Geometry check sheet. Reference: the model listing, model coordinates, mm. Face numbers are marked on the shaded views. A direction names the side the tool comes from. Round coordinates to 2 decimals unless told otherwise and drop trailing zeros. Write each loop counter-clockwise with the first axis right and the second up, starting at its lowest first coordinate (ties: lowest second). Pieces come first, ordered by that corner, then holes.
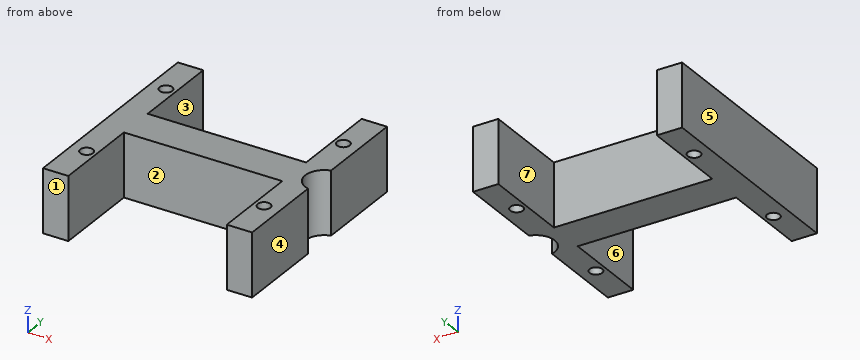
from build123d import *

# Parameters (mm, degrees)
CYLINDER156_R     = 3
CYLINDER156_DEPTH = 20
CYLINDER107_R     = 1
CYLINDER107_DEPTH = 15
CYLINDER108_R     = 1
CYLINDER108_DEPTH = 15
CYLINDER106_R     = 1
CYLINDER106_DEPTH = 15
CYLINDER105_R     = 1
CYLINDER105_DEPTH = 15
PAD005_DEPTH      = 10


with BuildPart() as zylinder156:
    # Cylinder156 → Cylinder156 (new body)
    with BuildSketch(Plane(origin=(28.75, 0, -21), x_dir=(1, 0, 0), z_dir=(0, 0, 1))):
        Circle(CYLINDER156_R)
    extrude(amount=CYLINDER156_DEPTH)


with BuildPart() as zylinder107:
    # Cylinder107 → Cylinder107 (new body)
    with BuildSketch(Plane(origin=(25.5, -10, -20), x_dir=(1, 0, 0), z_dir=(0, 0, 1))):
        Circle(CYLINDER107_R)
    extrude(amount=CYLINDER107_DEPTH)


with BuildPart() as zylinder108:
    # Cylinder108 → Cylinder108 (new body)
    with BuildSketch(Plane(origin=(25.5, 10, -20), x_dir=(1, 0, 0), z_dir=(0, 0, 1))):
        Circle(CYLINDER108_R)
    extrude(amount=CYLINDER108_DEPTH)


with BuildPart() as zylinder106:
    # Cylinder106 → Cylinder106 (new body)
    with BuildSketch(Plane(origin=(-2.5, -10, -20), x_dir=(1, 0, 0), z_dir=(0, 0, 1))):
        Circle(CYLINDER106_R)
    extrude(amount=CYLINDER106_DEPTH)


with BuildPart() as fusion074:
    # Cylinder105 → Cylinder105 (new body)
    with BuildSketch(Plane(origin=(-2.5, 10, -20), x_dir=(1, 0, 0), z_dir=(0, 0, 1))):
        Circle(CYLINDER105_R)
    extrude(amount=CYLINDER105_DEPTH)

    # Fusion074: union Zylinder107, Zylinder108, Zylinder106
    add(zylinder107.part)
    add(zylinder108.part)
    add(zylinder106.part)


with BuildPart() as fusion074_1:
    # Fusion074 placement: moved
    add(fusion074.part.moved(Location((0, 0, 17))))


with BuildPart() as cut076:
    # Sketch004 → Pad005 (new body)
    with BuildSketch(Plane.XY):
        Polygon((-5, 17), (-1, 17), (-1, 3), (24, 3), (24, 17), (28, 17), (28, -17), (24, -17), (24, -3), (-1, -3), (-1, -17), (-5, -17), align=None)
    extrude(amount=PAD005_DEPTH)

    # Cut055: cut Fusion074
    add(fusion074_1.part, mode=Mode.SUBTRACT)


with BuildPart() as cut076_1:
    # Cut055 placement: moved
    add(cut076.part.moved(Location((0, 0, -19))))

    # Cut076: cut Zylinder156
    add(zylinder156.part, mode=Mode.SUBTRACT)


solid = cut076_1.part
1. Release check for a two-part mould opening along X. For the marked faces 4, 5, 6 and 7 record: +X half, -X half, draft (parallel to the pull), parting line (faces both ways), or undercut.
2. Section check C-C (x = -2.5). Record the cut outline in (y, z).
3. Depth check by flat-ended pin: pin 1 Ø1 at (x, z) = (13, -13.5) entering from -Y. Enter the tip coordinate at first touch or a pass-through.
4. Scan lines: line 1 along Y through (x, z) = (25.5, -11.5); line 2 along X through (y, z) = (10, -13); line 3 along X through (y, z) = (13.5, -15). Record each from-to range of solid material in increasing order.
5. Section check D-D (x = 2). Record the cut outline in (y, z).
6. Section check A-A (y = -5.5). Record the cut outline in (x, z).
7. Access from +Z, -Z, +X, -X, +Y, -Y to the whole of each face (thin tool, end or side, straight path). Record for the marked faces 1, 2 and 3.
8. Section check B-B (z = -11.25). Record the cut outline in (x, y), plus the area to 3 significant figures.
Results below:
1. face 4: +X half
1. face 5: -X half
1. face 6: undercut
1. face 7: undercut
2. outline: (-17, -19) - (-11, -19) - (-11, -9) - (-17, -9) - close; (-9, -19) - (9, -19) - (9, -9) - (-9, -9) - close; (11, -19) - (17, -19) - (17, -9) - (11, -9) - close
3. pin 1: stops at y = -3
4. line 1: y = -17 to -11, -9 to 9, 11 to 17
4. line 2: x = -5 to -3.5, -1.5 to -1, 24 to 24.5, 26.5 to 28
4. line 3: x = -5 to -1, 24 to 28
5. outline: (-3, -19) - (3, -19) - (3, -9) - (-3, -9) - close
6. outline: (-5, -19) - (-1, -19) - (-1, -9) - (-5, -9) - close; (24, -19) - (28, -19) - (28, -9) - (24, -9) - close
7. face 1: +Z, -Z, +X, -X, -Y
7. face 2: +Z, -Z, -Y
7. face 3: +Z, -Z, +Y
8. outline: (-5, -17) - (-1, -17) - (-1, -3) - (24, -3) - (24, -17) - (28, -17) - (28, -2.9) arc R3 cw to (28, 2.9) - (28, 17) - (24, 17) - (24, 3) - (-1, 3) - (-1, 17) - (-5, 17) - close; hole circle Ø2 at (-2.5, -10); hole circle Ø2 at (-2.5, 10); hole circle Ø2 at (25.5, -10); hole circle Ø2 at (25.5, 10)
8. area: 400 mm2
